```python
from build123d import *

# Parameters (mm, degrees)
SKETCH1_R           = 14.2875
SKETCH1_R_2         = 9.398
BOSS_EXTRUDE2_DEPTH = 15.24
FILLET1_R           = 6.35


with BuildPart() as part:
    # Sketch1 → Boss-Extrude2 (new body)
    # profile 1 of 2: a face of its own
    with BuildSketch(Plane(origin=(0, 0, 0), x_dir=(1, 0, 0), z_dir=(0, 1, 0))):
        with BuildLine():
            ThreePointArc((9.525, -10.649273743), (-5.46758954, -13.199928821), (-14.265365769, -0.794981587))
            Line((-14.265365769, -0.794981587), (-60.194122004, -46.723737823))
            ThreePointArc((-60.194122004, -46.723737823), (-29.160477546, -70.399620377), (9.525, -75.602343714))
            Line((9.525, -75.602343714), (9.525, -10.649273743))
        make_face()
    # profile 2 of 2: a face of its own
    with BuildSketch(Plane(origin=(0, 0, 0), x_dir=(1, 0, 0), z_dir=(0, 1, 0))):
        Circle(SKETCH1_R)
        with Locations(Location((0, 0, 0), (0, 0, 90))):
            Circle(SKETCH1_R_2, mode=Mode.SUBTRACT)
    extrude(amount=BOSS_EXTRUDE2_DEPTH)

    # Fillet1
    fillet1_edges = [part.edges().sort_by_distance(p)[0] for p in [
        (9.525, 15.24, 43.125808728),
        (-37.229743887, 15.24, 23.759359705),
        (9.525, 0, 43.125808728),
        (-37.229743887, 0, 23.759359705),
    ]]
    fillet(fillet1_edges, radius=FILLET1_R)


solid = part.part
```
Source: CAD feature listing. Evaluate the final solid. Frame: model axes, mm. A direction names the side the tool comes from. Coordinates: 2 decimals unless noted, no trailing zeros. Order: outer loops, then holes, each group sorted by start corner. A loop starts at its lowest first (then second) coordinate and runs counter-clockwise, first axis right, second up. Notation, with made-up numbers: M 58.25,-39.5 L 105.25,-39.5 A22 cw 105.25,-24.5 Z; hole C -26.75,80 d11. An arc over 180 degrees is marked long. Write each question's results on one line, items separated by ' | '. Start each with the question number.
1) Section query D-D (z = 53.5). Return the cut outline in (x, y) (3 decimals), plus the area to 3 significant figures.
2) Draft query along X for faces 6 (the face through (-14, 15.24, 40)), 7 (the face through (-9.32, 7.51, 1.22)), 8 (the face through (5.93, 7.51, -13)). Return one class per face: released by +X, released by -X, zero draft, split by the parting line, or undercut.
3) Access query for faces 1 (the face through (-36.91, 7.6, 23.44)), 2 (the face through (9.525, 8, 44)), 3 (the face through (7.714, 1.91, 42.933)), 4 (the face through (7.615, 13.429, 42.933)), 5 (the face through (-14, 0, 40)). Directions: +Z, -Z, +X, -X, +Y, -Y. A direction counts if a zero-diameter tool reaches every point of the face in a straight line with its end or side. Return the directions, or none.
4) Section query C-C (y = 4). Return the cut outline in (x, z) (1 decimal).
5) Section query A-A (x = 0). Return the cut outline in (y, z).
6) Contact query for flat-ended pins moving along their axis: pin 1 Ø2 at (y, z) = (8, 59) entering from -X; pin 2 Ø4 at (y, z) = (2.5, -4) entering from -X; pin 3 Ø3 at (x, y) = (-52.5, 11) entering from +Z. Output: stop coordinate, or through.
7) Section query B-B (z = -3). Return the cut outline in (x, y).
8) Line query: line 1 (X direction, y = 7.5, z = 0); line 2 (Z direction, x = -3.5, y = 11.75); line 3 (Z direction, x = -6, y = 1.25). Output: solid intervals per line, ascending. Write a range as from..to.
Answers:
1) outline: M -54.26,0 L 3.175,0 A6.35 ccw 9.525,6.35 L 9.525,8.89 A6.35 ccw 3.175,15.24 L -54.26,15.24 Z | area: 955 mm^2
2) face 6: zero draft | face 7: undercut | face 8: split by the parting line
3) face 1: -Z, -X, +Y, -Y | face 2: +Z, +X, +Y, -Y | face 3: +Z, +X, -Y | face 4: +Z, +X, +Y | face 5: +Z, -Z, +X, -X, -Y
4) outline: M -59.9,47.1 L -14.2,1.4 A14.3 ccw long 9.1,11 L 9.1,75.7 A76.2 ccw Z; hole C 0,0 d18.8
5) outline: M 0,-14.29 L 15.24,-14.29 L 15.24,-9.4 L 0,-9.4 Z; M 0,9.4 L 15.24,9.4 L 15.24,76.2 L 0,76.2 Z
6) pin 1: stops at x = -49.42 | pin 2: stops at x = -14.15 | pin 3: stops at z = 56.62
7) outline: M -13.97,0 L -8.91,0 L -8.91,15.24 L -13.97,15.24 Z; M 8.91,0 L 13.97,0 L 13.97,15.24 L 8.91,15.24 Z
8) line 1: x = -14.29..-9.4, 9.4..14.29 | line 2: z = -13.85..-8.72, 8.72..76.12 | line 3: z = -12.97..-7.23, 7.23..75.96
